Can you work these out from the drawing? Everything is in mm from the part's minimum corner. A direction names the side the tool comes from. Round coordinates to 2 decimals unless told otherwise and drop trailing zeros. Loops run counter-clockwise (first coordinate to the right, second up) from the corner with the lowest first, then second, coordinate; pieces in that order, holes last. Notation, with made-up numbers: (16, -28) -> (73, -28) arc R23 ccw to (73, -1) -> close; hole circle Ø7 at (-37.5, -17.75). An arc over 180 degrees is marked (long way). Use CSV: the item, a comma, the result in double quotes. Start each with the question number.
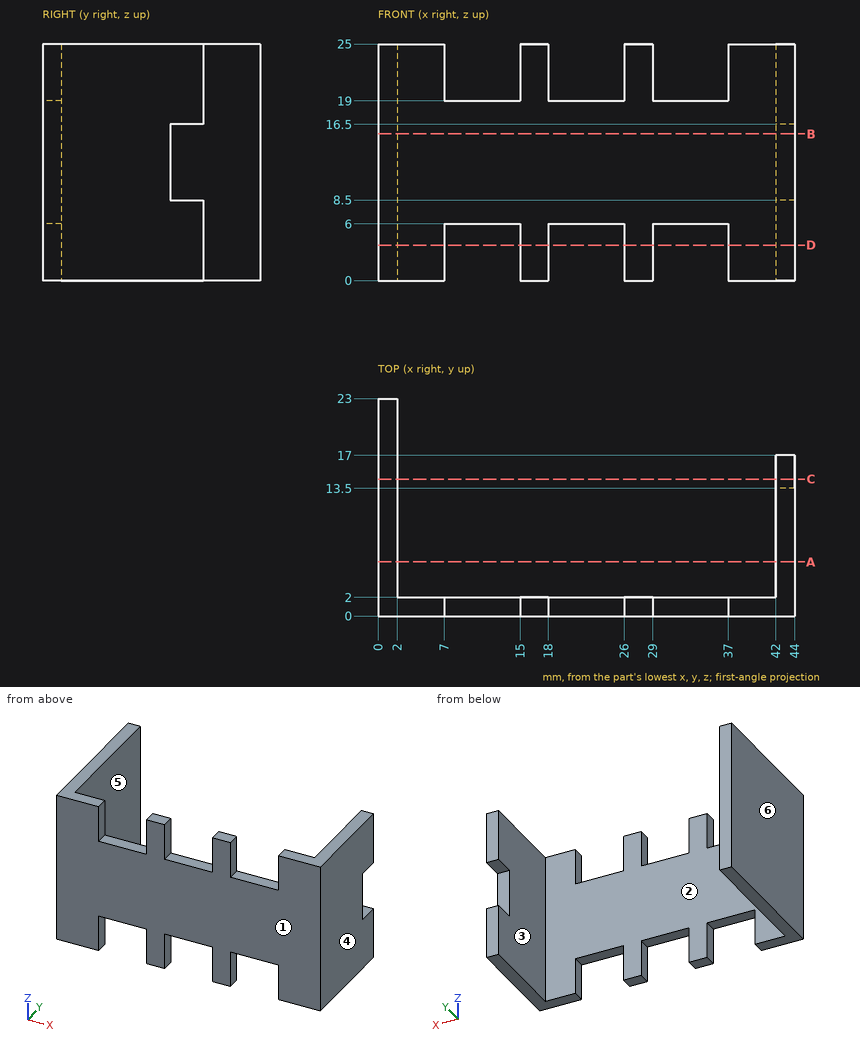
1. If I drill on L1, parallel to X at y = 10.75, z = 3.5; L2, parallel to Y at x = 23, z = 13, over which ranges is the centre line in solid material (lowest first)?
2. For the marked faces 1 and 2, which set-ups out of +Z, -Z, +X, -X, +Y, -Y let a thin tool reach every point of the face, with its end or its side?
3. We'd pull the mould along X, two halves only. Please class the marked faces 3, 4, 5 and 6: pulls with the +X half, pulls with the -X half, needs draft (parallel to the pull), parting line crosses it, or undercut.
4. Suppose I cut it at D-D (z = 3.75). List the corners of the cut face in (x, y) for me, then the cut area to 3 significant figures.
5. Suppose I cut it at B-B (z = 15.5). List the corners of the cut face in (x, y) for me.
6. Suppose I cut it at A-A (y = 5.75). List the corners of the cut face in (x, z) for me.
7. Will these pins go through, and if not, where does the flat tip stop? pin 1 (0.6 mm diameter, centred on x = 43, z = 5.5, fed in from +Y); pin 2 (1.6 mm diameter, centred on x = 22, y = 0.5, fed in from +Z); pin 3 (10.5 mm diameter, centred on y = 17.5, z = 18.5, fed in from +X); pin 4 (7.5 mm diameter, centred on x = 30.5, z = 9.5, fed in from +Y).
8. Suppose I cut it at C-C (y = 14.5). List the corners of the cut face in (x, z) for me, then the cut area to 3 significant figures.
Geometry check:
1,L1,"x = 0 to 2, 42 to 44"
1,L2,"y = 0 to 2"
2,face 1,"+Z, -Z, +X, -X, -Y"
2,face 2,"+Z, -Z, +Y"
3,face 3,"undercut"
3,face 4,"pulls with the +X half"
3,face 5,"undercut"
3,face 6,"pulls with the -X half"
4,outline,"(0, 0) -> (7, 0) -> (7, 2) -> (2, 2) -> (2, 23) -> (0, 23) -> close; (15, 0) -> (18, 0) -> (18, 2) -> (15, 2) -> close; (26, 0) -> (29, 0) -> (29, 2) -> (26, 2) -> close; (37, 0) -> (44, 0) -> (44, 17) -> (42, 17) -> (42, 2) -> (37, 2) -> close"
4,area,"112 mm²"
5,outline,"(0, 0) -> (44, 0) -> (44, 13.5) -> (42, 13.5) -> (42, 2) -> (2, 2) -> (2, 23) -> (0, 23) -> close"
6,outline,"(0, 0) -> (2, 0) -> (2, 25) -> (0, 25) -> close; (42, 0) -> (44, 0) -> (44, 25) -> (42, 25) -> close"
7,pin 1,"stops at y = 17"
7,pin 2,"stops at z = 19"
7,pin 3,"stops at x = 44"
7,pin 4,"stops at y = 2"
8,outline,"(0, 0) -> (2, 0) -> (2, 25) -> (0, 25) -> close; (42, 0) -> (44, 0) -> (44, 8.5) -> (42, 8.5) -> close; (42, 16.5) -> (44, 16.5) -> (44, 25) -> (42, 25) -> close"
8,area,"84.0 mm²"
